Design review of the part built by this model. Coordinates are the model's own, in mm. A direction names the side the tool comes from. Coordinates: 2 decimals unless noted, no trailing zeros. Loops run counter-clockwise (first coordinate to the right, second up) from the corner with the lowest first, then second, coordinate; pieces in that order, holes last. Notation, with made-up numbers: (-26.5, 61.25) - (12.5, 61.25) arc R19 ccw to (12.5, 85.25) - close; hole circle Ø8 at (52.5, 56.5). An arc over 180 degrees is marked (long way). Answer in a Markdown table with one row per item. Add a question column.
(1) To check wall thickness, follow L1, parallel to X at y = 2.95, z = -5 (3 decimals); L2, parallel to Y at x = 14.5, z = -8; L3, parallel to Z at x = 5, y = 1.5 (3 decimals). State the ranges of each line that lie inside material, in increasing order. Write a range as [from, to].
(2) Clearance check with flat-ended pins moving along their axes: pin 1 (5 mm diameter, centred on x = 30.5, z = -33.5, fed in from +Y); pin 2 (8.5 mm diameter, centred on x = 19, z = -7, fed in from +Y); pin 3 (8 mm diameter, centred on x = 15, z = -31, fed in from +Y); pin 4 (1.6 mm diameter, centred on x = 40, z = -5, fed in from +Y). State where each tip first meets the part, or that it passes through.
(3) We need section D-D, the plane y = 11.5. Write out the cut boundary in (x, z).
(4) The part is to be moulded in two halves that separate along Z. For faces 1 (the face through (44, 3, -43)), 2 (the face through (38.626, 3.042, -5.06)), 3 (the face through (45, 8, -22)), say which applies: released by +Z, released by -Z, zero draft, split by the parting line, or undercut.
(5) We need section A-A, the plane y = 2.5. Write out the cut boundary in (x, z) (3 decimals), plus the area to 3 significant figures.
(6) We need section C-C, the plane z = -33. Write out the cut boundary in (x, y).
(7) For faces 4 (the face through (23, 6, -5)), 5 (the face through (23, 6, -40)), 6 (the face through (0, 8, -23)), list the 3-axis set-ups (+Z, -Z, +X, -X, +Y, -Y) from which the entire face can be reached by the end or side of a thin tool; tool diameter is ignored.
Autodesk Inventor part; units mm, degrees
ref_plane "YZ Plane" through (0, 0, 0) normal (1, 0, 0) x (0, 1, 0)
ref_plane "XZ Plane" through (0, 0, 0) normal (0, 1, 0) x (-1, 0, 0)
ref_plane "XY Plane" through (0, 0, 0) normal (0, 0, 1) x (1, 0, 0)
sketch "Sketch1" plane through (0, 0, 0) normal (0, 1, 0) x (-1, 0, 0)
  line L0 (0, 0) -> (-45, 0)
  line L1 (-45, 0) -> (-45, -45)
  line L2 (-45, -45) -> (0, -45)
  line L3 (0, -45) -> (0, 0)
  dimension "d0" = 45
  dimension "d1" = 45
extrude "Extrusion1" add sketch "Sketch1" along normal blind 6
sketch "Sketch2" plane through (45, 0, 0) normal (1, 0, 0) x (0, 0, -1)
  line L0 (0, 0) -> (45, 0)
  line L1 (45, 0) -> (45, 6)
  line L2 (0, 6) -> (45, 6)
  line L3 (0, 0) -> (0, 6)
  line L4 (22.5, 0) -> (30.25, 0)
  line L5 (0, 0) -> (45, 0)
  line L6 (30.25, 0) -> (14.75, 0)
  line L7 (22.5, 0) -> (22.5, 6.5)
  arc A0 (30.25, 0) -> (14.75, 0) centre (22.5, -1.3702) ccw
  line L8 (14.75, 0) -> (8.75, 0)
  line L9 (30.25, 0) -> (36.25, 0)
  line L10 (22.5, 6.5) -> (22.5, 12.5)
  arc A1 (36.25, 0) -> (8.75, 0) centre (22.5, -1.3125) ccw
  arc A2 (30.25, 0) -> (14.75, 0) centre (22.5, -1.3702) ccw
  line L11 (14.75, 0) -> (30.25, 0)
  point P0 (22.5, 3)
  dimension "d4" = 7.75
  dimension "d5" = 15.5
  dimension "d6" = 6.5
  dimension "d7" = 6
  dimension "d8" = 6
  dimension "d9" = 6
extrude "Extrusion2" add sketch "Sketch2" against normal blind 45 contours A1 L2 A0 L0 | A1 L10 A0 L2 | A1 L2 A0 L10 | A0 L2 A1 L0
sketch "Sketch3" plane through (45, 0, 0) normal (1, 0, 0) x (0, 0, -1)
  line L0 (0, 0) -> (45, 0)
  line L1 (0, 6) -> (45, 6)
  line L2 (22.5, 0) -> (30.25, 0)
  line L3 (0, 0) -> (45, 0)
  line L4 (30.25, 0) -> (14.75, 0)
  line L5 (22.5, 0) -> (22.5, 6.5)
  arc A0 (30.25, 0) -> (14.75, 0) centre (22.5, -1.3702) ccw
  line L6 (14.75, 0) -> (8.75, 0)
  line L7 (30.25, 0) -> (36.25, 0)
  line L8 (22.5, 6.5) -> (22.5, 12.5)
  arc A1 (30.25, 0) -> (14.75, 0) centre (22.5, -1.3702) ccw
  line L9 (14.75, 0) -> (30.25, 0)
  point P0 (22.5, 3)
  point P1 (22.5, -1.3125)
  dimension "d12" = 7.75
  dimension "d13" = 15.5
  dimension "d14" = 6.5
  dimension "d15" = 6
  dimension "d16" = 6
  dimension "d17" = 6
extrude "Extrusion3" cut sketch "Sketch3" against normal blind 45
fillet "Fillet1" radius 5 4 edges at (45, 3, 0) (45, 3, -45) (0, 3, 0) (0, 3, -45)
sketch "Sketch4" plane through (0, 6, 0) normal (0, 1, 0) x (1, 0, 0)
  arc A0 (0, 5) -> (5, 0) centre (5, 5) ccw
  line L0 (5, 0) -> (40, 0)
  arc A1 (40, 0) -> (45, 5) centre (40, 5) ccw
  line L1 (45, 5) -> (45, 10.782)
  line L2 (45, 10.782) -> (0, 10.782)
  line L3 (0, 10.782) -> (0, 5)
  line L4 (45, 10.782) -> (0, 10.782)
  line L5 (45, 34.218) -> (45, 10.782)
  line L6 (0, 34.218) -> (45, 34.218)
  line L7 (0, 10.782) -> (0, 34.218)
  arc A2 (5, 45) -> (0, 40) centre (5, 40) ccw
  line L8 (0, 40) -> (0, 34.218)
  line L9 (0, 34.218) -> (45, 34.218)
  line L10 (45, 34.218) -> (45, 40)
  arc A3 (45, 40) -> (40, 45) centre (40, 40) ccw
  line L11 (40, 45) -> (5, 45)
  line L12 (5, 5) -> (5, 40)
  line L13 (5, 40) -> (40, 40)
  line L14 (40, 40) -> (40, 5)
  line L15 (40, 5) -> (5, 5)
  circle A4 centre (5, 5) radius 1.375
  circle A5 centre (40, 5) radius 1.375
  circle A6 centre (5, 40) radius 1.375
  circle A7 centre (40, 40) radius 1.375
  point P0 (0, 0)
  dimension "d21" = 2.75
  dimension "d22" = 2.75
  dimension "d23" = 2.75
  dimension "d24" = 2.75
extrude "Extrusion4" cut sketch "Sketch4" against normal blind 45 contours A4 L15 L12 | L12 L15 A4 | A5 L15 L14 | L14 L15 A5 | A6 L13 L12 | L12 L13 A6 | A7 L13 L14 | L14 L13 A7
sketch "Sketch5" plane through (0, 0, 0) normal (0, -1, 0) x (1, 0, 0)
  line L0 (45, -5) -> (45, -14.75)
  line L1 (45, -14.75) -> (45, -30.25)
  line L2 (45, -30.25) -> (45, -40)
  arc A0 (40, -45) -> (45, -40) centre (40, -40) ccw
  circle A1 centre (40, -40) radius 1.375
  circle A2 centre (40, -5) radius 1.375
  arc A3 (45, -5) -> (40, 0) centre (40, -5) ccw
  line L3 (5, 0) -> (40, 0)
  circle A4 centre (5, -5) radius 1.375
  arc A5 (5, 0) -> (0, -5) centre (5, -5) ccw
  line L4 (0, -14.75) -> (0, -5)
  line L5 (0, -30.25) -> (0, -14.75)
  line L6 (0, -40) -> (0, -30.25)
  arc A6 (0, -40) -> (5, -45) centre (5, -40) ccw
  line L7 (40, -45) -> (5, -45)
  circle A7 centre (5, -40) radius 1.375
  point P0 (0, 0)
properties part number "Roof" material "PC/ABS Plastic"
Responses:
| question | item | result |
|---|---|---|
| 1 | L1 | x = [0, 3.625], [6.375, 38.625], [41.375, 45] |
| 1 | L2 | y = [0, 6] |
| 1 | L3 | z = [-45, -41.375], [-38.625, -29.828], [-15.172, -6.375], [-3.625, 0] |
| 2 | pin 1 | stops at y = 9.57 |
| 2 | pin 2 | stops at y = 6.7 |
| 2 | pin 3 | stops at y = 11.75 |
| 2 | pin 4 | passes through |
| 3 | outline | (0, -27.66) - (45, -27.66) - (45, -17.34) - (0, -17.34) - close |
| 4 | face 1 | released by -Z |
| 4 | face 2 | undercut |
| 4 | face 3 | zero draft |
| 5 | outline | (0, -40) arc R5 ccw to (5, -45) - (40, -45) arc R5 ccw to (45, -40) - (45, -29.353) - (0, -29.353) - close; (0, -15.647) - (45, -15.647) - (45, -5) arc R5 ccw to (40, 0) - (5, 0) arc R5 ccw to (0, -5) - close; hole circle Ø2.75 at (5, -40); hole circle Ø2.75 at (5, -5); hole circle Ø2.75 at (40, -40); hole circle Ø2.75 at (40, -5) |
| 5 | area | 1,360 mm2 |
| 6 | outline | (0, 0) - (45, 0) - (45, 7.66) - (0, 7.66) - close |
| 7 | face 4 | +Z, +X, -X, +Y |
| 7 | face 5 | -Z, +X, -X, +Y |
| 7 | face 6 | +Z, -Z, -X, +Y, -Y |
